Study the drawing (mm; zero at the part's minimum x, y, z) and answer. Round coordinates to 2 decimals unless told otherwise and drop trailing zeros. Loops run counter-clockwise (first coordinate to the right, second up) from the corner with the lowest first, then second, coordinate; pieces in that order, holes last. Notation, with made-up numbers: (47.25, -32) -> (51.25, -32) arc R23 ccw to (51.25, -4) -> close; hole circle Ø10 at (62.5, 88.5). An arc over 180 degrees is marked (long way). Answer in a Markdown table with one row per item. Add a question column.
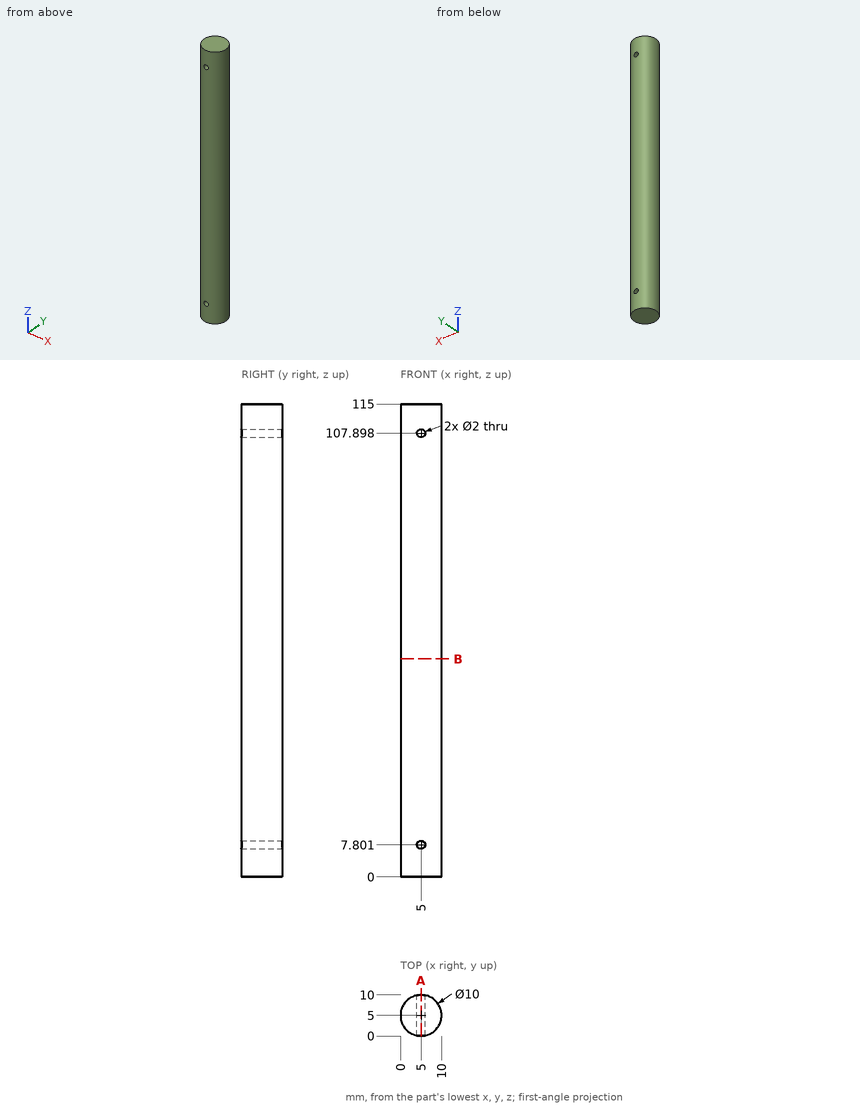
Item 1: Flat-ended cylindrical pins translate along their axes: P1, Ø1, axis at y = 7.5, z = 29.5, coming from the -X side; P2, Ø4, axis at x = 9, z = 95.5, coming from the -Y side; P3, Ø1.6, axis at x = 5, z = 107.9, coming from the -Y side; P4, Ø1, axis at y = 3, z = 65, coming from the -X side. Find the tip coordinate at first contact, or state that the pin passes through.
Item 2: Section A-A, the plane x = 5 is taken. Write down the section's boundary in (y, z).
Item 3: Section B-B, the plane z = 53 is taken. Write down the section's boundary in (x, y).
Item 4: Consider L1, parallel to Z at x = 4.75, y = 2; L2, parallel to Y at x = 5.25, z = 97; L3, parallel to Y at x = 2.75, z = 68.5 (1 decimal). Determine where each line is inside the solid, lowest interval first. Write a range as from..to.
Here are the results:
| question | item | result |
|---|---|---|
| 1 | P1 | stops at x = 0.42 |
| 1 | P2 | stops at y = 0.42 |
| 1 | P3 | passes through |
| 1 | P4 | stops at x = 0.23 |
| 2 | outline | (0, 0) -> (10, 0) -> (10, 6.8) -> (0, 6.8) -> close; (0, 8.8) -> (10, 8.8) -> (10, 106.9) -> (0, 106.9) -> close; (0, 108.9) -> (10, 108.9) -> (10, 115) -> (0, 115) -> close |
| 3 | outline | circle Ø10 at (5, 5) |
| 4 | L1 | z = 0..6.83, 8.77..106.93, 108.87..115 |
| 4 | L2 | y = 0.01..9.99 |
| 4 | L3 | y = 0.5..9.5 |
